Read the model definition and answer for the solid it produces. Units are mm, in the model's axes. A direction names the side the tool comes from. Round coordinates to 2 decimals unless told otherwise and drop trailing zeros. Order: outer loops, then holes, each group sorted by start corner. A loop starts at its lowest first (then second) coordinate and runs counter-clockwise, first axis right, second up. Notation, with made-up numbers: (-26.75, -23.75) -> (1.25, -23.75) arc R24 cw to (1.25, 8.25) -> close; hole circle Ø11 at (35, -19). An arc over 180 degrees is marked (long way). Use a Markdown table: item, result. Add a question column.
1. Consider L1, parallel to Z at x = 0, y = -11.9 (1 decimal); L2, parallel to X at y = 10.25, z = -43; L3, parallel to Y at x = 18.5, z = 27. Determine where each line is inside the solid, lowest interval first. Write a range as [from, to].
2. Section B-B, the plane y = 4 is taken. Give the vertices of the cut face in (x, z) (1 decimal).
3. The mould has two halves that part along Y. Classify faces 1 (the face through (-23.812, 0, -1)), 2 (the face through (0, -12.7, -1)), 3 (the face through (0, -11.112, -1)), 4 (the face through (-15.56, 11.92, -84.61)): +Y half, -Y half, draft (parallel to the pull), parting line (faces both ways), or undercut.
4. Section C-C, the plane x = -8 is taken. Give the vertices of the cut face in (y, z) (1 decimal).
5. Section D-D, the plane z = -70.5 is taken. Give the vertices of the cut face in (x, y), then the cut area to 3 significant figures.
6. For faces 5 (the face through (20.056, -11.917, -96.815)), 6 (the face through (24.6, -6.5, -88.9)), 7 (the face through (0, 11.112, -1)), determine the directions among +Z, -Z, +X, -X, +Y, -Y from which every point of the face is accessible in a straight line to the end or side of a thin tool.
7. Section A-A, the plane z = -38.1 is taken. Give the vertices of the cut face in (x, y).
8. Given pin 1 (6 mm diameter, centred on x = 6, y = -8.5, fed in from -Z) (3 decimals), flat-ended and moving along its own axis, determine where the tip first touches the part or whether it passes through.
```python
from build123d import *

# Parameters (mm, degrees)
BOSS_EXTRUDE1_DEPTH         = 98.424999
BOSS_EXTRUDE1_DEPTH_BACK    = 98.424999
SKETCH3_W                   = 50.8
SKETCH3_H                   = 25.4
SKETCH3_W_2                 = 47.625
SKETCH3_H_2                 = 22.225
SKETCH4_R                   = 14.2875
CUT_EXTRUDE3_DEPTH          = 105.774999061
CUT_EXTRUDE5_DEPTH          = 1.5875
CUT_EXTRUDE6_DEPTH          = 1.5875
F_10_CLEARANCE_HOLE1_D      = 4.9784
F_20_0_161_DIAMETER_HOLE1_D = 4.0894
F_20_0_161_DIAMETER_HOLE2_D = 4.0894


with BuildPart() as part:
    # Sketch3 → Boss-Extrude1 (new, two sides: drawn at the far end of the back side and taken through both)
    with BuildSketch(Plane.XY.offset(-BOSS_EXTRUDE1_DEPTH_BACK)):
        Rectangle(SKETCH3_W, SKETCH3_H)
        Rectangle(SKETCH3_W_2, SKETCH3_H_2, mode=Mode.SUBTRACT)
    extrude(amount=BOSS_EXTRUDE1_DEPTH + BOSS_EXTRUDE1_DEPTH_BACK)

    # Sketch4 → Cut-Extrude3 (cut, through all)
    with BuildSketch(Plane.XZ.offset(12.7)):
        with Locations((0, 73.025)):
            Circle(SKETCH4_R)
        with Locations((0, -73.025)):
            Circle(SKETCH4_R)
    extrude(amount=-CUT_EXTRUDE3_DEPTH, mode=Mode.SUBTRACT)

    # Sketch5 → Cut-Extrude5 (cut)
    with BuildSketch(Plane(origin=(25.4, 0, 0), x_dir=(0, 0, -1), z_dir=(1, 0, 0))):
        with BuildLine():
            Line((98.424999492, 0), (98.424999492, -12.7))
            Line((98.424999492, -12.7), (95.249999492, -12.7))
            ThreePointArc((95.249999492, -12.7), (88.899999492, -6.35), (95.249999492, 0))
            Line((95.249999492, 0), (98.424999492, 0))
        make_face()
    extrude(amount=-CUT_EXTRUDE5_DEPTH, mode=Mode.SUBTRACT)

    # Sketch6 → Cut-Extrude6 (cut)
    with BuildSketch(Plane.XZ.offset(12.7)):
        Polygon((23.8125, -98.424999492), (23.8125, -95.249999492), (16.1925, -98.424999492), align=None)
    extrude(amount=-CUT_EXTRUDE6_DEPTH, mode=Mode.SUBTRACT)

    # #10 Clearance Hole1 (through all)
    with Locations(Plane(origin=(0, -12.7, 0), x_dir=(-1, 0, 0), z_dir=(0, -1, 0))):
        with Locations((-19.05, 85.724999492), (19.05, 92.074999492), (19.05, 38.099999492), (-19.05, 38.099999492)):
            Hole(F_10_CLEARANCE_HOLE1_D / 2)

    # #20 (0.161) Diameter Hole1 (through all)
    with Locations(Plane(origin=(0, -12.7, 0), x_dir=(-1, 0, 0), z_dir=(0, -1, 0))):
        with Locations((15.293699364, 82.581564015), (-15.293699364, 63.468435985)):
            Hole(F_20_0_161_DIAMETER_HOLE1_D / 2)

    # #20 (0.161) Diameter Hole2 (through all)
    with Locations(Plane(origin=(0, 12.7, 0), x_dir=(1, 0, 0), z_dir=(0, 1, 0))):
        with Locations((-12.751963692, -60.273036308), (12.751963692, -85.776963692)):
            Hole(F_20_0_161_DIAMETER_HOLE2_D / 2)


solid = part.part
```
Verdict:
| question | item | result |
|---|---|---|
| 1 | L1 | z = [-98.4, -87.3], [-58.7, 58.7], [87.3, 98.4] |
| 1 | L2 | x = [-25.4, -23.81], [23.81, 25.4] |
| 1 | L3 | y = [-12.7, -11.11], [11.11, 12.7] |
| 2 | outline | (-25.4, -98.4) -> (-23.8, -98.4) -> (-23.8, 98.4) -> (-25.4, 98.4) -> close; (23.8, -98.4) -> (25.4, -98.4) -> (25.4, 98.4) -> (23.8, 98.4) -> close |
| 3 | face 1 | undercut |
| 3 | face 2 | -Y half |
| 3 | face 3 | undercut |
| 3 | face 4 | draft |
| 4 | outline | (-12.7, -98.4) -> (-11.1, -98.4) -> (-11.1, -84.9) -> (-12.7, -84.9) -> close; (-12.7, -61.2) -> (-11.1, -61.2) -> (-11.1, 61.2) -> (-12.7, 61.2) -> close; (-12.7, 84.9) -> (-11.1, 84.9) -> (-11.1, 98.4) -> (-12.7, 98.4) -> close; (11.1, -98.4) -> (12.7, -98.4) -> (12.7, -84.9) -> (11.1, -84.9) -> close; (11.1, -61.2) -> (12.7, -61.2) -> (12.7, 61.2) -> (11.1, 61.2) -> close; (11.1, 84.9) -> (12.7, 84.9) -> (12.7, 98.4) -> (11.1, 98.4) -> close |
| 5 | outline | (-25.4, -12.7) -> (-14.06, -12.7) -> (-14.06, -11.11) -> (-23.81, -11.11) -> (-23.81, 11.11) -> (-14.06, 11.11) -> (-14.06, 12.7) -> (-25.4, 12.7) -> close; (14.06, -12.7) -> (25.4, -12.7) -> (25.4, 12.7) -> (14.06, 12.7) -> (14.06, 11.11) -> (23.81, 11.11) -> (23.81, -11.11) -> (14.06, -11.11) -> close |
| 5 | area | 143 mm2 |
| 6 | face 5 | -Z, +X, -Y |
| 6 | face 6 | -Z, +X |
| 6 | face 7 | +Z, -Z |
| 7 | outline | (-25.4, -12.7) -> (-21.54, -12.7) -> (-21.54, -11.11) -> (-23.81, -11.11) -> (-23.81, 11.11) -> (-21.54, 11.11) -> (-21.54, 12.7) -> (-25.4, 12.7) -> close; (-16.56, -12.7) -> (16.56, -12.7) -> (16.56, -11.11) -> (-16.56, -11.11) -> close; (-16.56, 11.11) -> (16.56, 11.11) -> (16.56, 12.7) -> (-16.56, 12.7) -> close; (21.54, -12.7) -> (25.4, -12.7) -> (25.4, 12.7) -> (21.54, 12.7) -> (21.54, 11.11) -> (23.81, 11.11) -> (23.81, -11.11) -> (21.54, -11.11) -> close |
| 8 | pin 1 | stops at z = -98.425 |
